Autodesk Inventor part; units mm, degrees
ref_plane "Work Plane1" through (0, 0, 38.1) normal (0, 0, 1) x (1, 0, 0)
ref_plane "YZ Plane" through (0, 0, 0) normal (1, 0, 0) x (0, 1, 0)
ref_plane "XZ Plane" through (0, 0, 0) normal (0, 1, 0) x (-1, 0, 0)
sketch "Sketch1" plane through (0, 0, 0) normal (0, 0, 1) x (1, 0, 0)
  line L0 (0, 0) -> (-31.75, 0)
  line L1 (-31.75, 0) -> (-31.75, 1.5875)
  line L2 (-31.75, 1.5875) -> (0, 1.5875)
  line L3 (0, 1.5875) -> (0, 0)
  circle A0 centre (0, 4.7625) radius 4.7625
  circle A1 centre (0, 4.7625) radius 3.175
  dimension "d0" = 31.75
  dimension "d1" = 1.5875
  dimension "d2" = 9.525
  dimension "d3" = 6.35
extrude "Extrusion1" add sketch "Sketch1" along normal mid plane 127
ref_plane "Work Plane1" through (0, 0, 38.1) normal (0, 0, 1) x (1, 0, 0)
sketch "Sketch2" plane through (0, 0, 38.1) normal (0, 0, 1) x (1, 0, 0)
  arc A0 (0, 0) -> (-3.5498, 1.5875) centre (0, 4.7625) ccw
  line L0 (-3.5498, 1.5875) -> (-3.5498, 0)
  line L1 (-3.5498, 0) -> (0, 0)
extrude "Extrusion2" cut sketch "Sketch2" along normal blind 25.4
pattern_linear "Rectangular Pattern1" count 3 spacing 50.8 along (0, 0, -1) of "Extrusion2"
sketch "Sketch3" plane through (-31.75, 1.5875, -63.5) normal (0, 1, 0) x (1, 0, 0)
  line L0 (28.2002, 0) -> (0, 0) construction
  line L1 (0, -127) -> (28.2002, -127) construction
  line L2 (0, 0) -> (28.2002, 0) construction
  line L3 (28.2002, 0) -> (28.2002, -127) construction
  line L4 (28.2002, -127) -> (0, -127) construction
  line L5 (0, -127) -> (0, 0) construction
  line L6 (21.8502, -120.65) -> (21.8502, -6.35) construction
  line L7 (21.8502, -6.35) -> (6.35, -6.35) construction
  line L8 (6.35, -6.35) -> (6.35, -120.65) construction
  line L9 (6.35, -120.65) -> (21.8502, -120.65) construction
  line L10 (6.35, -82.55) -> (21.8502, -82.55) construction
  line L11 (6.35, -44.45) -> (21.8502, -44.45) construction
  line L12 (6.35, -6.35) -> (21.8502, -6.35) construction
  point P0 (31.75, -63.5)
  dimension "d12" = 6.35
  dimension "d15" = 114.3
hole "Hole1" at (-9.8998, 1.5875, -57.15) at (-25.4, 1.5875, 57.15) at (-9.8998, 1.5875, 19.05) at (-25.4, 1.5875, -19.05) direction (0, -1, 0) diameter 3.175 end through all
chamfer "Chamfer1" distance 0.7937 angle 45 4 edges at (-25.4, 1.5875, 55.5625) (-9.8998, 1.5875, 17.4625) (-25.4, 1.5875, -20.6375) (-9.8998, 1.5875, -58.7375)
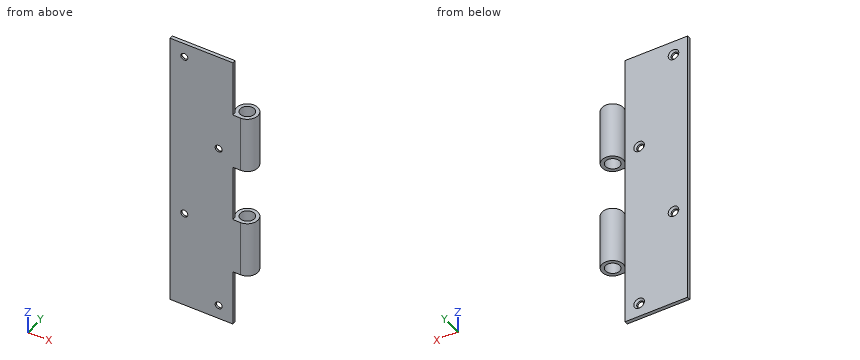
The listing builds one solid part. Answer for the finished solid, in the listing's coordinates (mm). Give positions to 0.01 mm unless a question says otherwise; leave off trailing zeros. Order: outer loops, then holes, each group sorted by start corner. A loop starts at its lowest first (then second) coordinate and runs counter-clockwise, first axis right, second up. Notation, with made-up numbers: (80.25, 3.25) -> (115.25, 3.25) arc R22 cw to (115.25, 39.25) -> close; hole circle Ø11 at (20.5, -5). An arc over 180 degrees is marked (long way). Answer as a JSON object with one key per item and string values. Group by question number.
Item 1: The part is cut by section B-B on z = 19.05. Give the number of separate pieces and of enclosed holes in the cut face, and give its area (3 significant figures).
Item 2: Flat-ended cylindrical pins translate along their axes: pin 1 (0.5 mm diameter, centred on y = 1, z = -3.5, fed in from +X); pin 2 (10 mm diameter, centred on x = -9, z = -3, fed in from +Y); pin 3 (1 mm diameter, centred on x = -6.5, y = 5, fed in from +Z); pin 4 (3.5 mm diameter, centred on x = -25.4, z = 57.15, fed in from +Y). Find the tip coordinate at first contact, or state that the pin passes through.
Item 3: The part is cut by section C-C on y = 3. Write down the section's boundary in (x, z).
Item 4: The part is cut by section A-A on z = 57.15. Write down the section's boundary in (x, y), and give its area (3 significant figures).
Item 5: The part is cut by section D-D on x = -17. Write down the section's boundary in (y, z).
Item 6: Consider L1, parallel to Z at x = -25.4, y = 0.4; L2, parallel to Y at x = 0, z = 27 (1 decimal); L3, parallel to X at y = 0.65, z = -57.15. Determine where each line is inside the solid, lowest interval first. Write a range as from..to.
Result set:
{
 "1": {"separate pieces": "2", "enclosed holes": "1", "area": "80.4 mm²"},
 "2": {"pin 1": "x = -3.55", "pin 2": "y = 1.59", "pin 3": "through", "pin 4": "y = 0.96"},
 "3": {"outline": "(-4.42, -38.1) -> (-2.64, -38.1) -> (-2.64, -12.7) -> (-4.42, -12.7) -> close; (-4.42, 12.7) -> (-2.64, 12.7) -> (-2.64, 38.1) -> (-4.42, 38.1) -> close; (2.64, -38.1) -> (4.42, -38.1) -> (4.42, -12.7) -> (2.64, -12.7) -> close; (2.64, 12.7) -> (4.42, 12.7) -> (4.42, 38.1) -> (2.64, 38.1) -> close"},
 "4": {"outline": "(-31.75, 0) -> (-26.99, 0) -> (-26.99, 0.79) -> (-27.78, 1.59) -> (-31.75, 1.59) -> close; (-23.81, 0) -> (-3.55, 0) -> (-3.55, 1.59) -> (-23.02, 1.59) -> (-23.81, 0.79) -> close", "area": "39.1 mm²"},
 "5": {"outline": "(0, -63.5) -> (1.59, -63.5) -> (1.59, 63.5) -> (0, 63.5) -> close"},
 "6": {"L1": "-63.5..-20.64, -17.46..55.56, 58.74..63.5", "L2": "0..1.6, 7.9..9.5", "L3": "-31.75..-11.49, -8.31..-3.55"}
}
